```python
from build123d import *

# Parameters (mm, degrees)
SKETCH2_R                = 63.5
SKETCH2_R_2              = 57.15
BOSS_EXTRUDE1_DEPTH      = 228.6
BOSS_EXTRUDE2_DEPTH      = 114.3
BOSS_EXTRUDE2_DEPTH_BACK = 114.3
SKETCH3_R                = 63.5
SKETCH3_R_2              = 57.15
SKETCH4_R                = 57.15
CUT_EXTRUDE1_DEPTH       = 330.466493124
SKETCH5_R                = 57.15
CUT_EXTRUDE2_DEPTH       = 264.352805317
CUT_EXTRUDE3_DEPTH       = 264.352805317
CUT_EXTRUDE3_DEPTH_BACK  = 264.352805317
SKETCH6_W                = 187.910276351
SKETCH6_H                = 55.092106145
SKETCH6_W_2              = 179.956402219
SKETCH6_H_2              = 52.109403346


with BuildPart() as part:
    # Sketch2 → Boss-Extrude1 (new body)
    with BuildSketch(Plane(origin=(0, 0, 0), x_dir=(1, 0, 0), z_dir=(0, 1, 0))):
        with Locations(Location((0, 0, 0), (0, 0, 270))):
            Circle(SKETCH2_R)
        with Locations(Location((0, 0, 0), (0, 0, 270))):
            Circle(SKETCH2_R_2, mode=Mode.SUBTRACT)
    extrude(amount=BOSS_EXTRUDE1_DEPTH)

    # Sketch3 → Boss-Extrude2 (add, two sides: drawn at the far end of the back side and taken through both)
    with BuildSketch(Plane(origin=(0, 0, 0), x_dir=(0, 0, -1), z_dir=(1, 0, 0)).offset(-BOSS_EXTRUDE2_DEPTH_BACK)):
        with Locations((0, 114.3)):
            Circle(SKETCH3_R)
        with Locations((0, 114.3)):
            Circle(SKETCH3_R_2, mode=Mode.SUBTRACT)
    extrude(amount=BOSS_EXTRUDE2_DEPTH + BOSS_EXTRUDE2_DEPTH_BACK)

    # Sketch4 → Cut-Extrude1 (cut, through all)
    with BuildSketch(Plane.ZY.offset(114.3)):
        with Locations(Location((0, 114.3, 0), (0, 0, 180))):
            Circle(SKETCH4_R)
    extrude(amount=-CUT_EXTRUDE1_DEPTH, mode=Mode.SUBTRACT)

    # Sketch5 → Cut-Extrude2 (cut, through all)
    with BuildSketch(Plane(origin=(0, 228.6, 0), x_dir=(1, 0, 0), z_dir=(0, 1, 0))):
        with Locations(Location((0, 0, 0), (0, 0, 270))):
            Circle(SKETCH5_R)
    extrude(amount=-CUT_EXTRUDE2_DEPTH, mode=Mode.SUBTRACT)

    # Sketch6 → Cut-Extrude3 (cut, two sides: drawn at the far end of the back side and taken through both)
    with BuildSketch(Plane(origin=(0, 0, 0), x_dir=(0, 0, -1), z_dir=(1, 0, 0)).offset(-CUT_EXTRUDE3_DEPTH_BACK)):
        with Locations((10.108048375, 211.696053073)):
            Rectangle(SKETCH6_W, SKETCH6_H)
        with Locations((6.131111309, 18.395298327)):
            Rectangle(SKETCH6_W_2, SKETCH6_H_2)
    extrude(amount=CUT_EXTRUDE3_DEPTH + CUT_EXTRUDE3_DEPTH_BACK, mode=Mode.SUBTRACT)


solid = part.part
```
The listing builds one solid part. Answer for the finished solid, in the listing's coordinates (mm). A direction names the side the tool comes from. Coordinates: 2 decimals unless noted, no trailing zeros. Loops run counter-clockwise (first coordinate to the right, second up) from the corner with the lowest first, then second, coordinate; pieces in that order, holes last. Notation, with made-up numbers: (57.5, 48.25) - (91.5, 48.25) arc R15 ccw to (91.5, 70.25) - close; hole circle Ø3 at (52.25, -2.5). An arc over 180 degrees is marked (long way). Use a Markdown table: item, result. Add a question column.
1) For faces 1 (the cylindrical face through (69.05, 117.09, 63.44)), 2 (the cylindrical face through (-71, 157, 47)), 3 (the cylindrical face through (-38.64, 164.26, -50.39)), determine the directions among +Z, -Z, +X, -X, +Y, -Y from which every point of the face is accessible in a straight line to the end or side of a thin tool.
2) The part is cut by section A-A, the plane z = 0. Give the vertices of the cut face in (x, y).
3) The part is cut by section C-C, the plane x = 22. Give the vertices of the cut face in (y, z), and give its area (3 significant figures).
4) Given pin 1 (2 mm diameter, centred on x = 74.5, z = 20, fed in from +Y); pin 2 (5 mm diameter, centred on x = -52.5, y = 138.5, fed in from -Z); pin 3 (6 mm diameter, centred on x = 79, y = 59.5, fed in from -Z), each flat-ended and moving along its own axis, determine where each tip first touches the part or whether it passes through.
5) Find the intervals of material crossed by line 1 (Z direction, x = 0, y = 82.5); line 2 (Y direction, x = -89, z = 0); line 3 (Y direction, x = 41, z = -49.5), in increasing order.
6) The part is cut by section B-B, the plane y = 129.5. Give the vertices of the cut face in (x, z).
7) The part is cut by section D-D, the plane x = -83. Give the vertices of the cut face in (y, z).
Here are the results:
| question | item | result |
|---|---|---|
| 1 | face 1 | +X |
| 1 | face 2 | -X |
| 1 | face 3 | +Y |
| 2 | outline | (-114.3, 50.8) - (-63.5, 50.8) - (-63.5, 44.45) - (-57.15, 44.45) - (-57.15, 57.15) - (-114.3, 57.15) - close; (-114.3, 171.45) - (-57.15, 171.45) - (-57.15, 184.15) - (-63.5, 184.15) - (-63.5, 177.8) - (-114.3, 177.8) - close; (57.15, 44.45) - (63.5, 44.45) - (63.5, 50.8) - (114.3, 50.8) - (114.3, 57.15) - (57.15, 57.15) - close; (57.15, 171.45) - (114.3, 171.45) - (114.3, 177.8) - (63.5, 177.8) - (63.5, 184.15) - (57.15, 184.15) - close |
| 3 | outline | (44.45, -59.57) - (92.3, -59.57) arc R63.5 ccw to (136.3, -59.57) - (184.15, -59.57) - (184.15, -52.75) - (136.3, -52.75) arc R57.15 cw to (92.3, -52.75) - (44.45, -52.75) - close; (44.45, 52.75) - (92.3, 52.75) arc R57.15 cw to (136.3, 52.75) - (184.15, 52.75) - (184.15, 59.57) - (136.3, 59.57) arc R63.5 ccw to (92.3, 59.57) - (44.45, 59.57) - close |
| 3 | area | 1,880 mm^2 |
| 4 | pin 1 | stops at y = 174.89 |
| 4 | pin 2 | stops at z = -59.68 |
| 4 | pin 3 | stops at z = -36.73 |
| 5 | line 1 | z = -63.5 to -57.15, 57.15 to 63.5 |
| 5 | line 2 | y = 50.8 to 57.15, 171.45 to 177.8 |
| 5 | line 3 | y = 74.53 to 85.74, 142.86 to 154.07 |
| 6 | outline | (-114.3, -61.65) - (-15.2, -61.65) arc R63.5 ccw to (15.2, -61.65) - (114.3, -61.65) - (114.3, -55.09) - (15.2, -55.09) arc R57.15 cw to (-15.2, -55.09) - (-114.3, -55.09) - close; (-114.3, 55.09) - (-15.2, 55.09) arc R57.15 cw to (15.2, 55.09) - (114.3, 55.09) - (114.3, 61.65) - (15.2, 61.65) arc R63.5 ccw to (-15.2, 61.65) - (-114.3, 61.65) - close |
| 7 | outline | circle Ø127 at (114.3, 0); hole circle Ø114.3 at (114.3, 0) |
